Could you check a few things on this model? Use its own coordinates, in mm. A direction names the side the tool comes from. Round coordinates to 2 decimals unless told otherwise and drop trailing zeros. Write each loop counter-clockwise with the first axis right and the second up, starting at its lowest first coordinate (ties: lowest second). Pieces come first, ordered by that corner, then holes. Notation, with made-up numbers: (9.25, 35) -> (53.25, 35) arc R15 ccw to (53.25, 51) -> close; hole circle Ø7 at (25, 52.25). An arc over 180 degrees is marked (long way). Answer in a Markdown table with one row per item. Add a question column.
```python
from build123d import *

# Parameters (mm, degrees)
BOSS_EXTRUDE3_DEPTH = 6.35
SKETCH2_R           = 2
CUT_EXTRUDE1_DEPTH  = 6.35
SKETCH3_W           = 44.45
SKETCH3_H           = 34.144934764
CUT_EXTRUDE2_DEPTH  = 6.35
BOSS_EXTRUDE5_DEPTH = 6.35
CUT_EXTRUDE3_DEPTH  = 6.35
CUT_EXTRUDE4_DEPTH  = 6.35
SKETCH8_R           = 2
CUT_EXTRUDE5_DEPTH  = 6.35


with BuildPart() as part:
    # Sketch1 → Boss-Extrude3 (new body)
    with BuildSketch(Plane(origin=(0, 0, 0), x_dir=(1, 0, 0), z_dir=(0, 1, 0))):
        with BuildLine():
            ThreePointArc((101.6, -161.144934764), (118.310930869, -149.307647617), (133.654639598, -135.744934764))
            Line((133.654639598, -135.744934764), (124.436872293, -135.744934764))
            Line((124.436872293, -135.744934764), (101.6, -135.744934764))
            Line((101.6, -135.744934764), (101.6, -161.144934764))
        make_face()
        with BuildLine():
            Line((146.05, -112.163363002), (146.05, -101.6))
            Line((146.05, -101.6), (101.6, -101.6))
            Line((101.6, -101.6), (101.6, -135.744934764))
            Line((101.6, -135.744934764), (124.436872293, -135.744934764))
            ThreePointArc((124.436872293, -135.744934764), (135.756435031, -124.424325787), (146.05, -112.163363002))
        make_face()
        with BuildLine():
            Line((152.4, -76.2), (152.4, -101.6))
            Line((152.4, -101.6), (157.687433266, -106.887433266))
            ThreePointArc((157.687433266, -106.887433266), (155.08800922, -110.62531083), (152.4, -114.3))
            ThreePointArc((152.4, -114.3), (143.428677452, -125.373300524), (133.654639598, -135.744934764))
            Line((133.654639598, -135.744934764), (190.5, -135.744934764))
            Line((190.5, -135.744934764), (240.876195248, -135.744934764))
            ThreePointArc((240.876195248, -135.744934764), (203.220744642, -110.47631512), (158.75, -101.6))
            Line((158.75, -101.6), (158.75, -76.2))
            Line((158.75, -76.2), (152.4, -76.2))
        make_face()
        with BuildLine():
            Line((146.05, -76.2), (152.4, -76.2))
            Line((152.4, -76.2), (152.4, -50.8))
            Line((152.4, -50.8), (190.076195248, -12.7))
            ThreePointArc((190.076195248, -12.7), (190.5, 0), (190.076195248, 12.7))
            Line((190.076195248, 12.7), (152.4, 50.8))
            Line((152.4, 50.8), (152.4, 76.2))
            Line((152.4, 76.2), (146.05, 76.2))
            Line((146.05, 76.2), (146.05, 6.35))
            Line((146.05, 6.35), (133.35, 6.35))
            Line((133.35, 6.35), (133.35, -6.35))
            Line((133.35, -6.35), (146.05, -6.35))
            Line((146.05, -6.35), (146.05, -76.2))
        make_face()
        with BuildLine():
            Line((157.687433266, -106.887433266), (152.4, -101.6))
            Line((152.4, -101.6), (152.4, -76.2))
            Line((152.4, -76.2), (146.05, -76.2))
            Line((146.05, -76.2), (146.05, -101.6))
            Line((146.05, -101.6), (146.05, -112.163363002))
            ThreePointArc((146.05, -112.163363002), (135.756435031, -124.424325787), (124.436872293, -135.744934764))
            Line((124.436872293, -135.744934764), (133.654639598, -135.744934764))
            ThreePointArc((133.654639598, -135.744934764), (143.428677452, -125.373300524), (152.4, -114.3))
            ThreePointArc((152.4, -114.3), (155.08800922, -110.62531083), (157.687433266, -106.887433266))
        make_face()
        with BuildLine():
            Line((101.6, 101.6), (146.05, 101.6))
            Line((146.05, 101.6), (146.05, 112.163363002))
            ThreePointArc((146.05, 112.163363002), (135.756435031, 124.424325787), (124.436872293, 135.744934764))
            Line((124.436872293, 135.744934764), (101.6, 135.744934764))
            Line((101.6, 135.744934764), (101.6, 101.6))
        make_face()
        with BuildLine():
            Line((124.436872293, 135.744934764), (133.654639598, 135.744934764))
            ThreePointArc((133.654639598, 135.744934764), (118.310930869, 149.307647617), (101.6, 161.144934764))
            Line((101.6, 161.144934764), (101.6, 135.744934764))
            Line((101.6, 135.744934764), (124.436872293, 135.744934764))
        make_face()
        with BuildLine():
            Line((146.05, 76.2), (152.4, 76.2))
            Line((152.4, 76.2), (152.4, 101.6))
            Line((152.4, 101.6), (157.687433266, 106.887433266))
            ThreePointArc((157.687433266, 106.887433266), (155.08800922, 110.62531083), (152.4, 114.3))
            ThreePointArc((152.4, 114.3), (143.428677452, 125.373300524), (133.654639598, 135.744934764))
            Line((133.654639598, 135.744934764), (124.436872293, 135.744934764))
            ThreePointArc((124.436872293, 135.744934764), (135.756435031, 124.424325787), (146.05, 112.163363002))
            Line((146.05, 112.163363002), (146.05, 101.6))
            Line((146.05, 101.6), (146.05, 76.2))
        make_face()
        with BuildLine():
            Line((152.4, 50.8), (190.076195248, 12.7))
            Line((190.076195248, 12.7), (240.876195248, 12.7))
            ThreePointArc((240.876195248, 12.7), (204.016770224, 40.811197813), (158.75, 50.8))
            Line((158.75, 50.8), (158.75, 76.2))
            Line((158.75, 76.2), (152.4, 76.2))
            Line((152.4, 76.2), (152.4, 50.8))
        make_face()
        with BuildLine():
            Line((152.4, -50.8), (152.4, -76.2))
            Line((152.4, -76.2), (158.75, -76.2))
            Line((158.75, -76.2), (158.75, -50.8))
            ThreePointArc((158.75, -50.8), (204.016770224, -40.811197813), (240.876195248, -12.7))
            Line((240.876195248, -12.7), (190.076195248, -12.7))
            Line((190.076195248, -12.7), (152.4, -50.8))
        make_face()
        with BuildLine():
            ThreePointArc((190.076195248, -12.7), (190.5, 0), (190.076195248, 12.7))
            Line((190.076195248, 12.7), (240.876195248, 12.7))
            Line((240.876195248, 12.7), (240.876195248, -12.7))
            Line((240.876195248, -12.7), (190.076195248, -12.7))
        make_face()
        with BuildLine():
            ThreePointArc((158.75, 101.6), (203.220744642, 110.47631512), (240.876195248, 135.744934764))
            Line((240.876195248, 135.744934764), (190.5, 135.744934764))
            Line((190.5, 135.744934764), (133.654639598, 135.744934764))
            ThreePointArc((133.654639598, 135.744934764), (143.428677452, 125.373300524), (152.4, 114.3))
            ThreePointArc((152.4, 114.3), (155.08800922, 110.62531083), (157.687433266, 106.887433266))
            Line((157.687433266, 106.887433266), (152.4, 101.6))
            Line((152.4, 101.6), (152.4, 76.2))
            Line((152.4, 76.2), (158.75, 76.2))
            Line((158.75, 76.2), (158.75, 101.6))
        make_face()
    extrude(amount=BOSS_EXTRUDE3_DEPTH)

    # Sketch2 → Cut-Extrude1 (cut)
    with BuildSketch(Plane(origin=(0, 6.35, 0), x_dir=(1, 0, 0), z_dir=(0, 1, 0))):
        with Locations((139.7, 0)):
            Circle(SKETCH2_R)
        with Locations((114.080664861, 142.381475953)):
            Circle(SKETCH2_R)
        with Locations((114.080664861, -142.381475953)):
            Circle(SKETCH2_R)
    extrude(amount=-CUT_EXTRUDE1_DEPTH, mode=Mode.SUBTRACT)

    # Sketch3 → Cut-Extrude2 (cut)
    with BuildSketch(Plane(origin=(0, 6.35, 0), x_dir=(1, 0, 0), z_dir=(0, 1, 0))):
        with Locations((123.825, 118.672467382)):
            Rectangle(SKETCH3_W, SKETCH3_H)
        with Locations((123.825, -118.672467382)):
            Rectangle(SKETCH3_W, SKETCH3_H)
    extrude(amount=-CUT_EXTRUDE2_DEPTH, mode=Mode.SUBTRACT)

    # Sketch4 → Boss-Extrude5 (add)
    with BuildSketch(Plane(origin=(0, 6.35, 0), x_dir=(1, 0, 0), z_dir=(0, 1, 0))):
        with BuildLine():
            Line((146.05, 135.744934764), (240.876195248, 135.744934764))
            ThreePointArc((240.876195248, 135.744934764), (170.089511185, 142.146873772), (101.6, 161.144934764))
            Line((101.6, 161.144934764), (133.654639598, 135.744934764))
            Line((133.654639598, 135.744934764), (146.05, 135.744934764))
        make_face()
        with BuildLine():
            ThreePointArc((101.6, -161.144934764), (170.089511185, -142.146873772), (240.876195248, -135.744934764))
            Line((240.876195248, -135.744934764), (146.05, -135.744934764))
            Line((146.05, -135.744934764), (133.654639598, -135.744934764))
            Line((133.654639598, -135.744934764), (101.6, -161.144934764))
        make_face()
    extrude(amount=-BOSS_EXTRUDE5_DEPTH)

    # Sketch6 → Cut-Extrude3 (cut)
    with BuildSketch(Plane(origin=(0, 6.35, 0), x_dir=(1, 0, 0), z_dir=(0, 1, 0))):
        with BuildLine():
            ThreePointArc((204.6037507, 30.046043954), (182.300238804, 38.083813069), (158.75, 40.811197813))
            Line((158.75, 40.811197813), (158.75, -40.811197813))
            ThreePointArc((158.75, -40.811197813), (182.300238804, -38.083813069), (204.6037507, -30.046043954))
            Line((204.6037507, -30.046043954), (204.6037507, 30.046043954))
        make_face()
    extrude(amount=-CUT_EXTRUDE3_DEPTH, mode=Mode.SUBTRACT)

    # Sketch7 → Cut-Extrude4 (cut)
    with BuildSketch(Plane(origin=(0, 6.35, 0), x_dir=(1, 0, 0), z_dir=(0, 1, 0))):
        with BuildLine():
            ThreePointArc((158.75, 104.775), (202.635785869, 112.774751554), (240.876195248, 135.744934764))
            ThreePointArc((240.876195248, 135.744934764), (203.220744642, 110.47631512), (158.75, 101.6))
            Line((158.75, 101.6), (158.75, 104.775))
        make_face()
        with BuildLine():
            Line((158.75, 50.8), (158.75, 47.625))
            ThreePointArc((158.75, 47.625), (203.371932866, 38.531106957), (240.876195248, 12.7))
            ThreePointArc((240.876195248, 12.7), (204.016770224, 40.811197813), (158.75, 50.8))
        make_face()
        with BuildLine():
            ThreePointArc((158.75, -47.625), (203.371932866, -38.531106957), (240.876195248, -12.7))
            ThreePointArc((240.876195248, -12.7), (204.016770224, -40.811197813), (158.75, -50.8))
            Line((158.75, -50.8), (158.75, -47.625))
        make_face()
        with BuildLine():
            Line((158.75, -104.775), (158.75, -101.6))
            ThreePointArc((158.75, -101.6), (203.220744642, -110.47631512), (240.876195248, -135.744934764))
            ThreePointArc((240.876195248, -135.744934764), (202.635785869, -112.774751554), (158.75, -104.775))
        make_face()
    extrude(amount=-CUT_EXTRUDE4_DEPTH, mode=Mode.SUBTRACT)

    # Sketch8 → Cut-Extrude5 (cut)
    with BuildSketch(Plane(origin=(0, 6.35, 0), x_dir=(1, 0, 0), z_dir=(0, 1, 0))):
        with Locations((217.3037507, 0)):
            Circle(SKETCH8_R)
    extrude(amount=-CUT_EXTRUDE5_DEPTH, mode=Mode.SUBTRACT)


solid = part.part
```
(1) Suppose I cut it at A-A, the plane x = 184. State how many separate pieces and enclosed holes the cut face has, then the cut area to 3 significant figures.
(2) Suppose I cut it at B-B, the plane x = 224. Please give me the cut outline in (y, z).
(3) I need wall thicknesses on L1, parallel to Z at x = 139.7, y = 2.75; L2, parallel to Z at x = 193, y = 1.5; L3, parallel to X at y = 3.5, z = 0. Which ranges of each line are inside material? Lowest first, please.
(4) Suppose I cut it at D-D, the plane z = 77. Please give me the cut outline in (x, y), then the cut area to 3 significant figures.
(5) If we mould it in two halves opening along X, with no side actions, what happens to faces 1 (the face through (158.75, 3, -1)), 2 (the face through (146.05, 3, -72)), 3 (the face through (158.75, 3, 77)), 4 (the face through (204.604, 3, 0))? For each: pulls with the +X half, pulls with the -X half, needs draft (parallel to the pull), parting line crosses it, or undercut.
(6) For P1, Ø3, axis at y = 2, z = -80.5, coming from the +X side; P2, Ø1.9, axis at x = 139, y = 2, coming from the +Z side; P3, Ø1.9, axis at y = 4.5, z = 56, coming from the -X side; P4, Ø3, axis at x = 217.3, z = 0, coming from the -Y side, each with a flat end and sliding along its axis, tell me the tip position at first contact or that it passes through.
(7) On a 3-axis mill with a long thin cutter (end or side, diameter ignored), from which of +Z, -Z, +X, -X, +Y, -Y can I reach the whole of each face in a straight line? I mean faces 5 (the face through (140, 3, 6.35)), 6 (the face through (202.048, 3.219, -112.555)), 7 (the face through (169.109, 3.219, 142.327)). Say none if no direction works.
Response:
| question | item | result |
|---|---|---|
| 1 | separate pieces | 4 |
| 1 | enclosed holes | 0 |
| 1 | area | 503 mm² |
| 2 | outline | (0, -136.11) -> (6.35, -136.11) -> (6.35, -123.27) -> (0, -123.27) -> close; (0, -27.11) -> (6.35, -27.11) -> (6.35, 27.11) -> (0, 27.11) -> close; (0, 123.27) -> (6.35, 123.27) -> (6.35, 136.11) -> (0, 136.11) -> close |
| 3 | L1 | -148.94 to -135.74, -6.35 to -2, 2 to 6.35, 135.74 to 148.94 |
| 3 | L2 | -138.66 to -109.58, -42.36 to -34.95, 34.95 to 42.36, 109.58 to 138.66 |
| 3 | L3 | 133.35 to 137.7, 141.7 to 158.75, 204.6 to 215.3, 219.3 to 240.88 |
| 4 | outline | (146.05, 0) -> (158.75, 0) -> (158.75, 6.35) -> (146.05, 6.35) -> close |
| 4 | area | 80.6 mm² |
| 5 | face 1 | undercut |
| 5 | face 2 | pulls with the -X half |
| 5 | face 3 | pulls with the +X half |
| 5 | face 4 | undercut |
| 6 | P1 | x = 158.75 |
| 6 | P2 | z = 149.38 |
| 6 | P3 | x = 146.05 |
| 6 | P4 | through |
| 7 | face 5 | -X, +Y, -Y |
| 7 | face 6 | +X, +Y, -Y |
| 7 | face 7 | +Z, +X, +Y, -Y |
